The listing builds one solid part. Answer for the finished solid, in the listing's coordinates (mm). A direction names the side the tool comes from. Round coordinates to 2 decimals unless told otherwise and drop trailing zeros. Write each loop counter-clockwise with the first axis right and the second up, starting at its lowest first coordinate (ties: lowest second). Pieces come first, ordered by that corner, then holes.
(1) Each of these flat-tipped pins is pushed along its axis until it touches: pin 1 Ø3 at (x, z) = (75, -36) entering from +Y; pin 2 Ø4 at (y, z) = (36, -67) entering from -X; pin 3 Ø1.7 at (x, z) = (30, -28.5) entering from +Y. Where does it stop, or does it pass through?
(2) Find the intervals of material crossed by probe 1 along Z at (x, y) = (138, 13.5); probe 2 along X at (y, z) = (11.5, -16); probe 3 along X at (y, z) = (1.2, -20), in increasing order.
(3) A cutting plane is placed at A-A, the plane x = 115. Give the vertices of the cut face in (y, z).
(4) The mould has two halves that part along Z. Classify faces 1 (the face through (95, 43, -2)), 2 (the face through (83, 21, -106)), 3 (the face through (70, 10, -36)): +Z half, -Z half, draft (parallel to the pull), parting line (faces both ways), or undercut.
(5) For faces 4 (the face through (0, 1, -53)), 5 (the face through (7, 23, -103)), 6 (the face through (22, 23, -96)), 7 (the face through (16.5, 25.1, -25.5)), determine the directions among +Z, -Z, +X, -X, +Y, -Y from which every point of the face is accessible in a straight line to the end or side of a thin tool.
(6) A cutting plane is placed at B-B, the plane y = 14.5. Give the number of separate pieces and of enclosed holes in the cut face, and give its area (3 significant figures).
from build123d import *

# Parameters (mm, degrees)
SKETCH1_W                                      = 166
SKETCH1_H                                      = 106
BOSS_EXTRUDE1_DEPTH                            = 43
SHELL1_T                                       = -3
SKETCH2_W                                      = 3
SKETCH2_H                                      = 100
BOSS_EXTRUDE2_DEPTH                            = 40
SKETCH3_R                                      = 10
CUT_EXTRUDE1_DEPTH                             = 3
SKETCH4_R                                      = 7.5
CUT_EXTRUDE3_DEPTH                             = 3
SKETCH5_W                                      = 3
SKETCH5_H                                      = 100
BOSS_EXTRUDE4_DEPTH                            = 40
SKETCH6_W                                      = 3
SKETCH6_H                                      = 40
CUT_EXTRUDE4_DEPTH                             = 20
CSK_FOR_2_FLAT_HEAD_MACHINE_SCREW1_D           = 2.4384
CSK_FOR_2_FLAT_HEAD_MACHINE_SCREW1_CSINK_D     = 4.3688
CSK_FOR_2_FLAT_HEAD_MACHINE_SCREW1_CSINK_ANGLE = 82
CSK_FOR_2_FLAT_HEAD_MACHINE_SCREW2_D           = 2.4384
CSK_FOR_2_FLAT_HEAD_MACHINE_SCREW2_CSINK_D     = 4.3688
CSK_FOR_2_FLAT_HEAD_MACHINE_SCREW2_CSINK_ANGLE = 82
BOSS_EXTRUDE6_DEPTH                            = 1.5
SKETCH17_W                                     = 7
SKETCH17_H                                     = 7
BOSS_EXTRUDE7_DEPTH                            = 40
SKETCH20_W                                     = 10
SKETCH20_H                                     = 10
BOSS_EXTRUDE8_DEPTH                            = 15
SKETCH21_W                                     = 10
SKETCH21_H                                     = 10
BOSS_EXTRUDE9_DEPTH                            = 15
SKETCH22_W                                     = 10
SKETCH22_H                                     = 10
BOSS_EXTRUDE10_DEPTH                           = 15
SKETCH23_W                                     = 10
SKETCH23_H                                     = 10
BOSS_EXTRUDE11_DEPTH                           = 15
SKETCH24_W                                     = 10
SKETCH24_H                                     = 10
BOSS_EXTRUDE12_DEPTH                           = 15
SKETCH25_W                                     = 10
SKETCH25_H                                     = 10
BOSS_EXTRUDE13_DEPTH                           = 15
SKETCH26_W                                     = 10
SKETCH26_H                                     = 10
BOSS_EXTRUDE14_DEPTH                           = 15
SKETCH27_W                                     = 10
SKETCH27_H                                     = 10
BOSS_EXTRUDE15_DEPTH                           = 15
SKETCH28_R                                     = 1.4
CUT_EXTRUDE5_DEPTH                             = 10
MIRROR4_COPY_1_SKETCH_W                        = 7
MIRROR4_COPY_1_SKETCH_H                        = 7
MIRROR4_COPY_1_DEPTH                           = 40
MIRROR4_COPY_2_SKETCH_R                        = 1.4
MIRROR4_COPY_2_DEPTH                           = 10
FILLET2_R                                      = 2
FILLET3_R                                      = 2
SKETCH29_R                                     = 1.4
CUT_EXTRUDE6_DEPTH                             = 10
MIRROR6_COPY_1_SKETCH_R                        = 1.4
MIRROR6_COPY_1_DEPTH                           = 10
SKETCH30_R                                     = 1.4
CUT_EXTRUDE7_DEPTH                             = 10
SKETCH31_R                                     = 1.4
CUT_EXTRUDE8_DEPTH                             = 10
SKETCH32_R                                     = 1.4
CUT_EXTRUDE9_DEPTH                             = 10


with BuildPart() as part:
    # Sketch1 → Boss-Extrude1 (new body)
    with BuildSketch(Plane(origin=(0, 0, 0), x_dir=(1, 0, 0), z_dir=(0, 1, 0))):
        with Locations((83, 53)):
            Rectangle(SKETCH1_W, SKETCH1_H)
    extrude(amount=BOSS_EXTRUDE1_DEPTH)

    # Shell1
    shell1_openings = [part.faces().sort_by_distance(p)[0] for p in [
        (83, 43, -53),
        (166, 21.5, -53),
        (0, 21.5, -53),
    ]]
    offset(amount=SHELL1_T, openings=shell1_openings, kind=Kind.INTERSECTION)

    # Sketch2 → Boss-Extrude2 (add)
    with BuildSketch(Plane(origin=(0, 3, 0), x_dir=(1, 0, 0), z_dir=(0, 1, 0))):
        with Locations((16.5, 53)):
            Rectangle(SKETCH2_W, SKETCH2_H)
    extrude(amount=BOSS_EXTRUDE2_DEPTH)

    # Sketch3 → Cut-Extrude1 (cut)
    with BuildSketch(Plane.ZY.offset(-15)):
        with Locations((-86, 20)):
            Circle(SKETCH3_R)
    extrude(amount=-CUT_EXTRUDE1_DEPTH, mode=Mode.SUBTRACT)

    # Sketch4 → Cut-Extrude3 (cut)
    with BuildSketch(Plane.ZY.offset(-15)):
        with Locations((-20, 20)):
            Circle(SKETCH4_R)
    extrude(amount=-CUT_EXTRUDE3_DEPTH, mode=Mode.SUBTRACT)

    # Sketch5 → Boss-Extrude4 (add)
    with BuildSketch(Plane(origin=(0, 3, 0), x_dir=(1, 0, 0), z_dir=(0, 1, 0))):
        with Locations((144.5, 53)):
            Rectangle(SKETCH5_W, SKETCH5_H)
    extrude(amount=BOSS_EXTRUDE4_DEPTH)

    # Sketch6 → Cut-Extrude4 (cut)
    with BuildSketch(Plane(origin=(166, 0, 0), x_dir=(0, 0, -1), z_dir=(1, 0, 0))):
        with Locations((104.5, 23)):
            Rectangle(SKETCH6_W, SKETCH6_H)
    cut_extrude4 = extrude(amount=-CUT_EXTRUDE4_DEPTH, mode=Mode.SUBTRACT)

    # Mirror1: Cut-Extrude4 across plane
    add(cut_extrude4.mirror(Plane(origin=(0, 0, -53), x_dir=(1, 0, 0), z_dir=(0, 0, -1))), mode=Mode.SUBTRACT)

    # CSK for #2 Flat Head Machine Screw1 (through all)
    with Locations(Plane(origin=(156, 3, -86), x_dir=(0, 0, 1), z_dir=(0, 1, 0))):
        with Locations((0, 0), (66, 0)):
            CounterSinkHole(CSK_FOR_2_FLAT_HEAD_MACHINE_SCREW1_D / 2, CSK_FOR_2_FLAT_HEAD_MACHINE_SCREW1_CSINK_D / 2, counter_sink_angle=CSK_FOR_2_FLAT_HEAD_MACHINE_SCREW1_CSINK_ANGLE)

    # CSK for #2 Flat Head Machine Screw2 (through all)
    with Locations(Plane(origin=(0, 3, 0), x_dir=(1, 0, 0), z_dir=(0, 1, 0))):
        with Locations((7.5, 20), (7.5, 86)):
            CounterSinkHole(CSK_FOR_2_FLAT_HEAD_MACHINE_SCREW2_D / 2, CSK_FOR_2_FLAT_HEAD_MACHINE_SCREW2_CSINK_D / 2, counter_sink_angle=CSK_FOR_2_FLAT_HEAD_MACHINE_SCREW2_CSINK_ANGLE)

    # Sketch16 → Boss-Extrude6 (add, symmetric)
    with BuildSketch(Plane(origin=(0, 0, -96), x_dir=(-1, 0, 0), z_dir=(0, 0, -1))):
        Polygon((-153.8156, 3), (-146, 7.512338764), (-146, 3), align=None)
    boss_extrude6 = extrude(amount=BOSS_EXTRUDE6_DEPTH, both=True)

    # Mirror2: Boss-Extrude6 across plane
    add(boss_extrude6.mirror(Plane(origin=(0, 0, -53), x_dir=(1, 0, 0), z_dir=(0, 0, -1))))

    # Sketch17 → Boss-Extrude7 (add)
    with BuildSketch(Plane(origin=(0, 3, 0), x_dir=(1, 0, 0), z_dir=(0, 1, 0))):
        with Locations((139.5, 99.5)):
            Rectangle(SKETCH17_W, SKETCH17_H)
    boss_extrude7 = extrude(amount=BOSS_EXTRUDE7_DEPTH)

    # Sketch20 → Boss-Extrude8 (add)
    with BuildSketch(Plane(origin=(0, 3, 0), x_dir=(1, 0, 0), z_dir=(0, 1, 0))):
        with Locations((138, 91)):
            Rectangle(SKETCH20_W, SKETCH20_H)
    extrude(amount=BOSS_EXTRUDE8_DEPTH)

    # Sketch21 → Boss-Extrude9 (add)
    with BuildSketch(Plane(origin=(0, 3, 0), x_dir=(1, 0, 0), z_dir=(0, 1, 0))):
        with Locations((30, 28.5)):
            Rectangle(SKETCH21_W, SKETCH21_H)
    extrude(amount=BOSS_EXTRUDE9_DEPTH)

    # Sketch22 → Boss-Extrude10 (add)
    with BuildSketch(Plane(origin=(0, 3, 0), x_dir=(1, 0, 0), z_dir=(0, 1, 0))):
        with Locations((64, 12.5)):
            Rectangle(SKETCH22_W, SKETCH22_H)
    extrude(amount=BOSS_EXTRUDE10_DEPTH)

    # Sketch23 → Boss-Extrude11 (add)
    with BuildSketch(Plane(origin=(0, 3, 0), x_dir=(1, 0, 0), z_dir=(0, 1, 0))):
        with Locations((50, 86)):
            Rectangle(SKETCH23_W, SKETCH23_H)
    extrude(amount=BOSS_EXTRUDE11_DEPTH)

    # Sketch24 → Boss-Extrude12 (add)
    with BuildSketch(Plane(origin=(0, 3, 0), x_dir=(1, 0, 0), z_dir=(0, 1, 0))):
        with Locations((50, 41)):
            Rectangle(SKETCH24_W, SKETCH24_H)
    extrude(amount=BOSS_EXTRUDE12_DEPTH)

    # Sketch25 → Boss-Extrude13 (add)
    with BuildSketch(Plane(origin=(0, 3, 0), x_dir=(1, 0, 0), z_dir=(0, 1, 0))):
        with Locations((138, 36)):
            Rectangle(SKETCH25_W, SKETCH25_H)
    extrude(amount=BOSS_EXTRUDE13_DEPTH)

    # Sketch26 → Boss-Extrude14 (add)
    with BuildSketch(Plane(origin=(0, 3, 0), x_dir=(1, 0, 0), z_dir=(0, 1, 0))):
        with Locations((75, 91)):
            Rectangle(SKETCH26_W, SKETCH26_H)
    extrude(amount=BOSS_EXTRUDE14_DEPTH)

    # Sketch27 → Boss-Extrude15 (add)
    with BuildSketch(Plane(origin=(0, 3, 0), x_dir=(1, 0, 0), z_dir=(0, 1, 0))):
        with Locations((75, 36)):
            Rectangle(SKETCH27_W, SKETCH27_H)
    extrude(amount=BOSS_EXTRUDE15_DEPTH)

    # Sketch28 → Cut-Extrude5 (cut)
    with BuildSketch(Plane(origin=(0, 43, 0), x_dir=(1, 0, 0), z_dir=(0, 1, 0))):
        with Locations((141, 101)):
            Circle(SKETCH28_R)
    cut_extrude5 = extrude(amount=-CUT_EXTRUDE5_DEPTH, mode=Mode.SUBTRACT)

    # Mirror3: Boss-Extrude7, Cut-Extrude5 across plane
    add(boss_extrude7.mirror(Plane(origin=(0, 0, -53), x_dir=(1, 0, 0), z_dir=(0, 0, -1))))
    add(cut_extrude5.mirror(Plane(origin=(0, 0, -53), x_dir=(1, 0, 0), z_dir=(0, 0, -1))), mode=Mode.SUBTRACT)

    # Mirror4: Boss-Extrude7, Cut-Extrude5 across plane
    add(boss_extrude7.mirror(Plane.ZY.offset(-80.5)))
    add(cut_extrude5.mirror(Plane.ZY.offset(-80.5)), mode=Mode.SUBTRACT)

    # Mirror4 copy 1 sketch → Mirror4 copy 1 (add)
    with BuildSketch(Plane(origin=(161, 3, -106), x_dir=(-1, 0, 0), z_dir=(0, 1, 0))):
        with Locations((139.5, 99.5)):
            Rectangle(MIRROR4_COPY_1_SKETCH_W, MIRROR4_COPY_1_SKETCH_H)
    extrude(amount=MIRROR4_COPY_1_DEPTH)

    # Mirror4 copy 2 sketch → Mirror4 copy 2 (cut)
    with BuildSketch(Plane(origin=(161, 43, -106), x_dir=(-1, 0, 0), z_dir=(0, 1, 0))):
        with Locations((141, 101)):
            Circle(MIRROR4_COPY_2_SKETCH_R)
    extrude(amount=-MIRROR4_COPY_2_DEPTH, mode=Mode.SUBTRACT)

    # Fillet2
    fillet2_edges = [part.edges().sort_by_distance(p)[0] for p in [
        (146, 23, -106),
        (0, 21.5, -106),
        (0, 21.5, 0),
        (146, 23, 0),
    ]]
    fillet(fillet2_edges, radius=FILLET2_R)

    # Fillet3
    fillet3_edges = [part.edges().sort_by_distance(p)[0] for p in [
        (156, 3, 0),
        (156, 3, -106),
        (166, 3, -53),
    ]]
    fillet(fillet3_edges, radius=FILLET3_R)

    # Sketch29 → Cut-Extrude6 (cut)
    with BuildSketch(Plane(origin=(0, 18, 0), x_dir=(1, 0, 0), z_dir=(0, 1, 0))):
        with Locations((138, 91)):
            Circle(SKETCH29_R)
    cut_extrude6 = extrude(amount=-CUT_EXTRUDE6_DEPTH, mode=Mode.SUBTRACT)

    # Mirror5: Cut-Extrude6 across plane
    add(cut_extrude6.mirror(Plane(origin=(0, 0, -63.5), x_dir=(1, 0, 0), z_dir=(0, 0, -1))), mode=Mode.SUBTRACT)

    # Mirror6: Cut-Extrude6 across plane
    add(cut_extrude6.mirror(Plane.ZY.offset(-106.5)), mode=Mode.SUBTRACT)

    # Mirror6 copy 1 sketch → Mirror6 copy 1 (cut)
    with BuildSketch(Plane(origin=(213, 18, -127), x_dir=(-1, 0, 0), z_dir=(0, 1, 0))):
        with Locations((138, 91)):
            Circle(MIRROR6_COPY_1_SKETCH_R)
    extrude(amount=-MIRROR6_COPY_1_DEPTH, mode=Mode.SUBTRACT)

    # Sketch30 → Cut-Extrude7 (cut)
    with BuildSketch(Plane(origin=(0, 18, 0), x_dir=(1, 0, 0), z_dir=(0, 1, 0))):
        with Locations((50, 86)):
            Circle(SKETCH30_R)
    cut_extrude7 = extrude(amount=-CUT_EXTRUDE7_DEPTH, mode=Mode.SUBTRACT)

    # Mirror7: Cut-Extrude7 across plane
    add(cut_extrude7.mirror(Plane.XY.offset(-63.5)), mode=Mode.SUBTRACT)

    # Sketch31 → Cut-Extrude8 (cut)
    with BuildSketch(Plane(origin=(0, 18, 0), x_dir=(1, 0, 0), z_dir=(0, 1, 0))):
        with Locations((64, 12.5)):
            Circle(SKETCH31_R)
    extrude(amount=-CUT_EXTRUDE8_DEPTH, mode=Mode.SUBTRACT)

    # Sketch32 → Cut-Extrude9 (cut)
    with BuildSketch(Plane(origin=(0, 18, 0), x_dir=(1, 0, 0), z_dir=(0, 1, 0))):
        with Locations((30, 28.5)):
            Circle(SKETCH32_R)
    extrude(amount=-CUT_EXTRUDE9_DEPTH, mode=Mode.SUBTRACT)


solid = part.part
Solutions:
1. pin 1: stops at y = 18
1. pin 2: stops at x = 15
1. pin 3: stops at y = 8
2. probe 1: z = -106 to -92.4, -89.6 to -86, -41 to -37.4, -34.6 to -31, -10 to 0
2. probe 2: x = 15 to 18, 59 to 69, 143 to 146
2. probe 3: x = 0 to 6.28, 8.72 to 154.78, 157.22 to 165.99
3. outline: (0, -106) - (43, -106) - (43, -103) - (3, -103) - (3, -3) - (43, -3) - (43, 0) - (0, 0) - close
4. face 1: draft
4. face 2: -Z half
4. face 3: undercut
5. face 4: +Z, -Z, -X, +Y, -Y
5. face 5: -X, +Y
5. face 6: +Y
5. face 7: -X
6. separate pieces: 8
6. enclosed holes: 8
6. area: 2,340 mm2
